```python
from build123d import *

# Parameters (mm, degrees)
BOSS_EXTRU_1_DEPTH                                 = 20
ESQUISSE9_W                                        = 25
ESQUISSE9_H                                        = 100
BOSS_EXTRU_2_DEPTH                                 = 5
CHAMBRAGE_POUR_VIS_T_TE_HEXAGONALE_M53_D           = 5.5
CHAMBRAGE_POUR_VIS_T_TE_HEXAGONALE_M53_CBORE_D     = 10
CHAMBRAGE_POUR_VIS_T_TE_HEXAGONALE_M53_CBORE_DEPTH = 5
CHAMBRAGE_POUR_VIS_T_TE_HEXAGONALE_M54_D           = 5.5
CHAMBRAGE_POUR_VIS_T_TE_HEXAGONALE_M54_CBORE_D     = 10
CHAMBRAGE_POUR_VIS_T_TE_HEXAGONALE_M54_CBORE_DEPTH = 5
TROU_TARAUD_M52_D                                  = 4.2


with BuildPart() as part:
    # Esquisse1 → Boss.-Extru.1 (new body)
    with BuildSketch(Plane.XY):
        with BuildLine():
            Line((-225, 50), (-225, -50))
            Line((-225, -50), (-209.105236663, -50))
            ThreePointArc((-209.105236663, -50), (-215, 0), (-209.105236663, 50))
            Line((-209.105236663, 50), (-225, 50))
        make_face()
    extrude(amount=BOSS_EXTRU_1_DEPTH)

    # Esquisse9 → Boss.-Extru.2 (add)
    with BuildSketch(Plane.XY.offset(20)):
        with Locations((-212.5, 0)):
            Rectangle(ESQUISSE9_W, ESQUISSE9_H)
    extrude(amount=BOSS_EXTRU_2_DEPTH)

    # Chambrage pour vis à tête hexagonale M53 (through all)
    with Locations(Plane.ZY.offset(225)):
        with Locations((16, 35)):
            CounterBoreHole(CHAMBRAGE_POUR_VIS_T_TE_HEXAGONALE_M53_D / 2, CHAMBRAGE_POUR_VIS_T_TE_HEXAGONALE_M53_CBORE_D / 2, CHAMBRAGE_POUR_VIS_T_TE_HEXAGONALE_M53_CBORE_DEPTH)

    # Chambrage pour vis à tête hexagonale M54 (through all)
    with Locations(Plane.ZY.offset(225)):
        with Locations((16, -35)):
            CounterBoreHole(CHAMBRAGE_POUR_VIS_T_TE_HEXAGONALE_M54_D / 2, CHAMBRAGE_POUR_VIS_T_TE_HEXAGONALE_M54_CBORE_D / 2, CHAMBRAGE_POUR_VIS_T_TE_HEXAGONALE_M54_CBORE_DEPTH)

    # Trou taraudé M52 (through all)
    with Locations(Plane.ZY.offset(225)):
        with Locations((12.5, 20), (12.5, -20)):
            Hole(TROU_TARAUD_M52_D / 2)


solid = part.part
```
Design review of the part built by this model. Coordinates are the model's own, in mm. A direction names the side the tool comes from. Round coordinates to 2 decimals unless told otherwise and drop trailing zeros. Write each loop counter-clockwise with the first axis right and the second up, starting at its lowest first coordinate (ties: lowest second). Pieces come first, ordered by that corner, then holes. Notation, with made-up numbers: (36.25, -29) -> (41.25, -29) arc R20 ccw to (41.25, 0) -> close; hole circle Ø7 at (46, 79.25). An arc over 180 degrees is marked (long way). Answer in a Markdown table with one row per item.
Q1. Clearance check with flat-ended pins moving along their axes: pin 1 Ø3 at (y, z) = (34.5, 14) entering from -X; pin 2 Ø5 at (y, z) = (20, 12.5) entering from +X; pin 3 Ø12 at (y, z) = (-36.5, 17) entering from -X; pin 4 Ø7.5 at (x, y) = (-207.5, 8) entering from -Z. State where each tip first meets the part, or that it passes through.
The answers:
| item | result |
|---|---|
| pin 1 | x = -220 |
| pin 2 | x = -213.82 |
| pin 3 | x = -225 |
| pin 4 | z = 20 |
Q2. Take a section at A-A, the plane y = 35. State the section outline as (x, z) points.
The answers:
| item | result |
|---|---|
| outline | (-225, 0) -> (-212.13, 0) -> (-212.13, 13.25) -> (-220, 13.25) -> (-220, 11) -> (-225, 11) -> close; (-225, 21) -> (-220, 21) -> (-220, 18.75) -> (-212.13, 18.75) -> (-212.13, 20) -> (-200, 20) -> (-200, 25) -> (-225, 25) -> close |
Q3. To check wall thickness, follow L1, parallel to Y at x = -217.5, z = 12.5; L2, parallel to Y at x = -221.25, z = 16; L3, parallel to Z at x = -217.75, y = -35. State the ranges of each line that lie inside material, in increasing order. Write a range as [from, to].
The answers:
| item | result |
|---|---|
| L1 | [-50, -22.1], [-17.9, 17.9], [22.1, 50] |
| L2 | [-50, -40], [-30, 30], [40, 50] |
| L3 | [0, 13.25], [18.75, 25] |
Q4. Take a section at D-D, the plane x = -210. State the section outline as (y, z) points, then the cut area to 3 significant figures.
The answers:
| item | result |
|---|---|
| outline | (-50, 0) -> (-46.1, 0) -> (-46.1, 20) -> (46.1, 20) -> (46.1, 0) -> (50, 0) -> (50, 25) -> (-50, 25) -> close |
| area | 656 mm² |
Q5. Draft analysis for pull direction Y (two halves, no side actions). For faces 1 (the face through (-206, 1, 20)), 2 (the face through (-213, 1, 25)), 3 (the face through (-215, -50, 12)), state which applies: +Y half, -Y half, draft (parallel to the pull), parting line (faces both ways), or undercut.
The answers:
| item | result |
|---|---|
| face 1 | undercut |
| face 2 | draft |
| face 3 | -Y half |
Q6. For faces 4 (the face through (-220, 32.8, 18.2)), 5 (the face through (-215, -0.7, 9.9)), 6 (the face through (-215, 50, 12)), list the 3-axis set-ups (+Z, -Z, +X, -X, +Y, -Y) from which the entire face can be reached by the end or side of a thin tool; tool diameter is ignored.
The answers:
| item | result |
|---|---|
| face 4 | -X |
| face 5 | -Z, +X |
| face 6 | +Z, -Z, +X, -X, +Y |
Q7. Take a section at B-B, the plane x = -222. State the section outline as (y, z) points.
The answers:
| item | result |
|---|---|
| outline | (-50, 0) -> (50, 0) -> (50, 25) -> (-50, 25) -> close; hole circle Ø10 at (-35, 16); hole circle Ø4.2 at (-20, 12.5); hole circle Ø4.2 at (20, 12.5); hole circle Ø10 at (35, 16) |
Q8. Take a section at C-C, the plane z = 8.5. State the section outline as (x, y) points, then the cut area to 3 significant figures.
The answers:
| item | result |
|---|---|
| outline | (-225, -50) -> (-209.11, -50) arc R215 cw to (-209.11, 50) -> (-225, 50) -> close |
| area | 1,200 mm² |
